Verification items for the finished model (mm, model axes). Face numbers are marked on the shaded views. A direction names the side the tool comes from. Coordinates: 2 decimals unless noted, no trailing zeros. Write each loop counter-clockwise with the first axis right and the second up, starting at its lowest first coordinate (ties: lowest second). Pieces come first, ordered by that corner, then holes.
```python
from build123d import *

# Parameters (mm, degrees)
F0_W     = 206.834365
F0_H     = 91.075212
F1_DEPTH = 127
F2_DEPTH = 127
F3_R     = 38.508072
F3_R_2   = 39.324103
F4_DEPTH = 63.5
F5_W     = 100.627238
F5_H     = 15.888504
F6_DEPTH = 25.4


with BuildPart() as f1:
    # F0 (on Front) → F1 (new body)
    with BuildSketch(Plane.XZ):
        with Locations((41.707343, 0.141859)):
            Rectangle(F0_W, F0_H)
    extrude(amount=F1_DEPTH)

    # F0 (on Front) → F2 (join)
    with BuildSketch(Plane.XZ):
        with Locations((41.707343, 0.141859)):
            Rectangle(F0_W, F0_H)
    extrude(amount=F2_DEPTH)

    # F3 (on face) → F4 (cut)
    with BuildSketch(Plane.XZ.offset(127)):
        with Locations((-15.331196, 0)):
            Circle(F3_R)
        with Locations((94.186038, 0)):
            Circle(F3_R_2)
    extrude(amount=-F4_DEPTH, mode=Mode.SUBTRACT)

    # F5 (on face) → F6 (cut)
    with BuildSketch(Plane.XY.offset(45.679465)):
        with Locations((38.056093, -107.49064)):
            Rectangle(F5_W, F5_H)
    extrude(amount=-F6_DEPTH, mode=Mode.SUBTRACT)


solid = f1.part
```
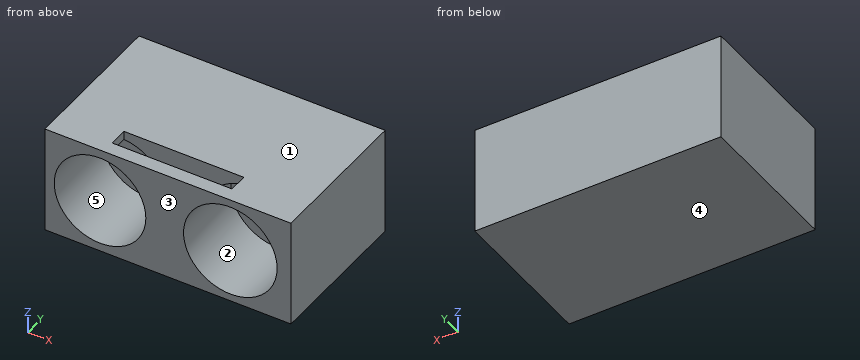
1. Sectioned sample at D-D, the plane z = 0. Record the boundary of the cut face in (x, y).
2. Material ranges on L1, parallel to X at y = -71, z = -24; L2, parallel to Z at x = 85.5, y = -76.5; L3, parallel to Y at x = -41, z = -26, recorded low to high.
3. Sectioned sample at C-C, the plane x = 38.5. Record the boundary of the cut face in (y, z), and give its area (3 significant figures).
4. Gauge pin test, flat ends, axial feed: P1, Ø8, axis at x = 3.5, z = 19, coming from the -Y side; P2, Ø8, axis at x = 31, y = -108.5, coming from the +Z side. Record the tip position at first contact, or that the pin passes through.
5. Draft check along Z on the marked faces 3, 4 and 5. Enter one of: pulls with the +Z half, pulls with the -Z half, needs draft (parallel to the pull), parting line crosses it, or undercut.
6. Sectioned sample at A-A, the plane y = -75. Record the boundary of the cut face in (x, z), and give its area (3 significant figures).
7. Tool access check on the marked faces 1 and 2. Record the directions out of +Z, -Z, +X, -X, +Y, -Y that give a thin tool (end or side, any length) a straight path to the whole face; none if there is none.
8. Sectioned sample at B-B, the plane x = -5.5. Record the boundary of the cut face in (y, z).
Outcome:
1. outline: (-61.71, -127) - (-53.84, -127) - (-53.84, -63.5) - (23.18, -63.5) - (23.18, -127) - (54.86, -127) - (54.86, -63.5) - (133.51, -63.5) - (133.51, -127) - (145.12, -127) - (145.12, 0) - (-61.71, 0) - close
2. L1: x = -61.71 to -45.45, 14.78 to 63.04, 125.34 to 145.12
2. L2: z = -45.4 to -38.35, 38.35 to 45.68
2. L3: y = -63.5 to 0
3. outline: (-127, -45.4) - (0, -45.4) - (0, 45.68) - (-99.55, 45.68) - (-99.55, 20.28) - (-115.43, 20.28) - (-115.43, 45.68) - (-127, 45.68) - close
3. area: 11,200 mm2
4. P1: stops at y = -63.5
4. P2: stops at z = 20.28
5. face 3: needs draft
5. face 4: pulls with the -Z half
5. face 5: undercut
6. outline: (-61.71, -45.4) - (145.12, -45.4) - (145.12, 45.68) - (-61.71, 45.68) - close; hole circle Ø77.02 at (-15.33, 0); hole circle Ø78.65 at (94.19, 0)
6. area: 9,320 mm2
7. face 1: +Z, +X, -X, +Y, -Y
7. face 2: -Y
8. outline: (-127, -45.4) - (0, -45.4) - (0, 45.68) - (-99.55, 45.68) - (-99.55, 37.23) - (-63.5, 37.23) - (-63.5, -37.23) - (-127, -37.23) - close; (-127, 37.23) - (-115.43, 37.23) - (-115.43, 45.68) - (-127, 45.68) - close
